Input: part model. Units: mm. Frame: model coordinates. A direction names the side the tool comes from. Round coordinates to 2 decimals unless told otherwise and drop trailing zeros. Loops run counter-clockwise (first coordinate to the right, second up) from the corner with the lowest first, then second, coordinate; pieces in that order, holes last. Notation, with made-up numbers: (-29, 62) - (26, 62) arc R21 cw to (26, 82) - close; hole circle Ø11 at (-31, -27.5). An arc over 180 degrees is marked (long way). Use CSV: the item, a comma, the result in double quotes. Start each with the question number.
1. Cut plane A-A (x = 7.5). Return loops of the section in (y, z), and give its area (3 significant figures).
2. Access query for faces 4 (the cylindrical face through (-0.487, 24.899, -23.206)), 5 (the flat face through (-3, 24.384, -1)). Directions: +Z, -Z, +X, -X, +Y, -Y. A direction counts if a zero-diameter tool reaches every point of the face in a straight line with its end or side. Return the directions, or none.
3. Cut plane D-D (x = 0). Give the number of separate pieces and of enclosed holes in the cut face, and give its area (3 significant figures).
4. Pin query (flat end, axial travel): P1, Ø6, axis at x = 0, z = 25.4, coming from the +Y side. Return the tip coordinate at first contact, or that it passes through.
5. Cut plane B-B (y = 11). Return loops of the section in (x, z), and give its area (3 significant figures).
6. Material intervals for probe 1 along Z at (x, y) = (0, 25.1); probe 2 along Y at (x, z) = (-2.5, -18); probe 3 along X at (y, z) = (-21.5, 31.5), sorted ascending. Write a range as from..to.
7. Cut plane C-C (z = -44.5). Return loops of the section in (x, y).
8. Pull-direction query (Y, two-part tool) for faces 1 (the cylindrical face through (2.076, 24.899, 0.861)), 2 (the flat face through (3, -24.384, -1)), 3 (the flat face through (-3, 25.4, -1)); classes: +Y half, -Y half, draft (parallel to the pull), parting line (faces both ways), or undercut.
Autodesk Inventor part; units mm, degrees
ref_plane "YZ Plane" through (0, 0, 0) normal (1, 0, 0) x (0, 1, 0)
ref_plane "XZ Plane" through (0, 0, 0) normal (0, 1, 0) x (-1, 0, 0)
ref_plane "XY Plane" through (0, 0, 0) normal (0, 0, 1) x (1, 0, 0)
sketch "Sketch1" plane through (0, 0, 0) normal (0, 0, 1) x (1, 0, 0)
  line L0 (12.7, 25.4) -> (-12.7, 25.4)
  line L1 (-12.7, 25.4) -> (-12.7, -25.4)
  line L2 (-12.7, -25.4) -> (12.7, -25.4)
  line L3 (12.7, -25.4) -> (12.7, 25.4)
  line L4 (12.7, 25.4) -> (-12.7, -25.4) construction
  line L5 (-12.7, 25.4) -> (12.7, -25.4) construction
  line L6 (-11.684, 24.384) -> (11.684, 24.384)
  line L7 (11.684, 24.384) -> (11.684, -24.384)
  line L8 (11.684, -24.384) -> (-11.684, -24.384)
  line L9 (-11.684, -24.384) -> (-11.684, 24.384)
  point P0 (0, 0)
  dimension "d0" = 1.016
  dimension "d1" = 50.8
  dimension "d2" = 25.4
extrude "Tube Length" add sketch "Sketch1" along normal mid plane 127
sketch "Sketch2" plane through (-12.7, 25.4, 63.5) normal (0, 1, 0) x (1, 0, 0)
  line L0 (0, 0) -> (0, 127)
  line L1 (25.4, 0) -> (0, 0)
  line L2 (25.4, 127) -> (25.4, 0)
  line L3 (0, 127) -> (25.4, 127)
  line L4 (25.4, 0) -> (0, 0)
  line L5 (12.7, 0) -> (12.7, 12.7) construction
  circle A0 centre (12.7, 12.7) radius 2.2479
  point P0 (12.7, 63.5)
  dimension "d5" = 12.7
  dimension "d6" = 4.4958
extrude "Top Hole" cut sketch "Sketch2" against normal through all contours A0
pattern_linear "Rectangular Pattern1" count 5 spacing 25.4 along (0, 0, -1) of "Top Hole"
sketch "Sketch3" plane through (0, 0, 63.5) normal (0, 0, 1) x (1, 0, 0)
  line L0 (0, 0) -> (0, 25.4) construction
  line L1 (12.7, 25.4) -> (-12.7, 25.4)
  line L2 (-0.0508, 25.4) -> (0, 25.2984)
  line L3 (0.0508, 25.4) -> (0, 25.2984)
  line L4 (-12.7, 12.6492) -> (-12.5984, 12.7)
  line L5 (-12.7, 12.7508) -> (-12.5984, 12.7)
  line L6 (-12.7, -0.0508) -> (-12.5984, 0)
  line L7 (-12.7, 0.0508) -> (-12.5984, 0)
  line L8 (-12.7, -12.7508) -> (-12.5984, -12.7)
  line L9 (-12.7, -12.6492) -> (-12.5984, -12.7)
  line L10 (12.7, 0.0508) -> (12.5984, 0)
  line L11 (12.7, 12.6492) -> (12.5984, 12.7)
  line L12 (12.7, 12.7508) -> (12.5984, 12.7)
  line L13 (12.7, -0.0508) -> (12.5984, 0)
  line L14 (12.7, -12.6492) -> (12.5984, -12.7)
  line L15 (12.7, -12.7508) -> (12.5984, -12.7)
  line L16 (0.0508, -25.4) -> (0, -25.2984)
  line L17 (-0.0508, -25.4) -> (0, -25.2984)
  line L18 (-12.7, 25.4) -> (-12.7, -25.4)
  line L19 (12.7, -25.4) -> (12.7, 25.4)
  line L20 (-12.7, -25.4) -> (12.7, -25.4)
  point P0 (0, 12.7)
  point P1 (-12.7, 12.7)
  point P2 (-12.7, 0)
  point P3 (-12.7, -12.7)
  point P4 (12.7, 12.7)
  point P5 (12.7, 0)
  point P6 (12.7, -12.7)
  point P7 (0, -25.4)
  dimension "d12" = 0.1016
  dimension "d13" = 0.1016
  dimension "d16" = 90
  dimension "d20" = 12.7
  dimension "d27" = 360
equation "\"d13\" = d12"
properties part number "Carrage Base & Top Tube" material "Aluminum 6061"
Established:
1,outline,"(-25.4, -63.5) - (-24.38, -63.5) - (-24.38, 63.5) - (-25.4, 63.5) - close; (24.38, -63.5) - (25.4, -63.5) - (25.4, 63.5) - (24.38, 63.5) - close"
1,area,"258 mm2"
2,face 4,"+Y, -Y"
2,face 5,"+Z, -Z"
3,separate pieces,"12"
3,enclosed holes,"0"
3,area,"212 mm2"
4,P1,"stops at y = 25.4"
5,outline,"(-12.7, -63.5) - (-11.68, -63.5) - (-11.68, 63.5) - (-12.7, 63.5) - close; (11.68, -63.5) - (12.7, -63.5) - (12.7, 63.5) - (11.68, 63.5) - close"
5,area,"258 mm2"
6,probe 1,"z = -63.5..-53.05, -48.55..-27.65, -23.15..-2.25, 2.25..23.15, 27.65..48.55, 53.05..63.5"
6,probe 2,"y = -25.4..-24.38, 24.38..25.4"
6,probe 3,"x = -12.7..-11.68, 11.68..12.7"
7,outline,"(-12.7, -25.4) - (12.7, -25.4) - (12.7, 25.4) - (-12.7, 25.4) - close; hole (-11.68, -24.38) - (11.68, -24.38) - (11.68, 24.38) - (-11.68, 24.38) - close"
8,face 1,"draft"
8,face 2,"undercut"
8,face 3,"+Y half"
